The drawing under review shows one solid part. Ordinate dimensions are in mm from its lowest x, y, z. Give positions to 0.01 mm unless a question says otherwise; leave off trailing zeros. Order: outer loops, then holes, each group sorted by start corner. A loop starts at its lowest first (then second) coordinate and runs counter-clockwise, first axis right, second up. Notation, with made-up numbers: (6, 15) - (18, 15) arc R23 cw to (18, 43) - close; hole circle Ø8 at (46, 75.5). An arc over 180 degrees is marked (long way). Write item = value, one per line. Start each with the question number.
1. For P1, Ø8, axis at x = 33, z = 8.5, coming from the -Y side; P2, Ø3, axis at y = 69, z = 14, coming from the -X side; P3, Ø10, axis at y = 47, z = 16.5, coming from the -X side, all flat-tipped, find the tip position at first contact; note any pin that passes through.
2. Mouldability with a two-part tool opening along X and no side actions: class the marked faces 1, 2 and 3 as pulls with the +X half, pulls with the -X half, needs draft (parallel to the pull), parting line crosses it, or undercut.
3. We need section A-A, the plane z = 2.25. Give the boundary of the cut face in (x, y) (1 decimal), and give its area (3 significant figures).
4. Wall thickness on probe 1 along Y at (x, z) = (36.5, 5.5); probe 2 along X at (y, z) = (43, 20.75); probe 3 along Y at (x, z) = (34.5, 5): over which ranges is each line inside the solid? List them lowest first.
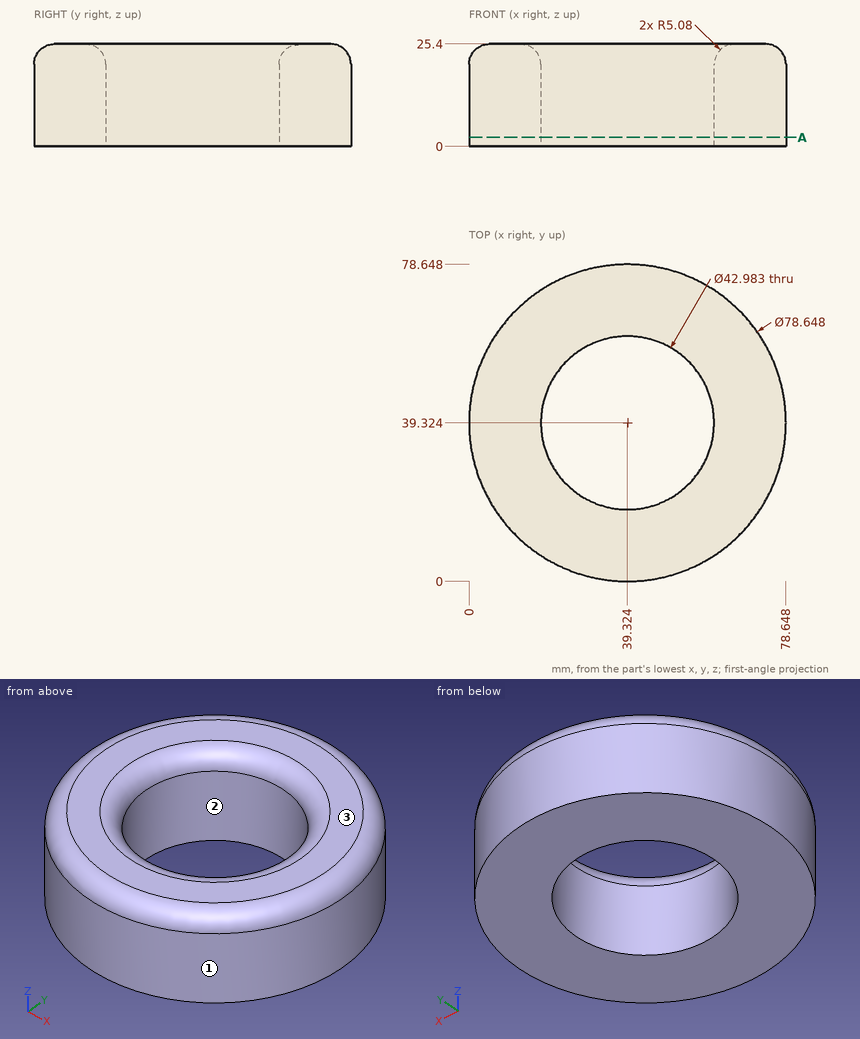
Model answer:
q1.P1 = 0.07
q1.P2 = 11.89
q1.P3 = 0.09
q2.face_1 = parting line crosses it
q2.face_2 = undercut
q2.face_3 = needs draft
q3.outline = circle Ø78.6 at (39.3, 39.3); hole circle Ø43 at (39.3, 39.3)
q3.area = 3,410 mm2
q4.probe_1 = 0.1 to 18.02, 60.63 to 78.55
q4.probe_2 = 0.19 to 18.13, 60.52 to 78.46
q4.probe_3 = 0.3 to 18.38, 60.27 to 78.35
